from build123d import *

# Parameters (mm, degrees)
CUT_EXTRUDE1_START    = -16
CUT_EXTRUDE1_DEPTH    = 16
F_3_0MM_DOWEL_HOLE1_D = 3
CUT_EXTRUDE3_START    = -20
SKETCH17_R            = 5
SKETCH17_R_2          = 4
CUT_EXTRUDE3_DEPTH    = 1.5
CHAMFER2_SIZE         = 1
THREAD2_PITCH         = 1


with BuildPart() as part:
    # Sketch1 → Revolve1 (revolve)
    with BuildSketch(Plane.XY, mode=Mode.PRIVATE) as revolve1_sk:
        Polygon((0, 0), (0, 5), (45, 5), (45, 4), (60, 4), (60, 0), align=None)
    revolve(revolve1_sk.sketch.rotate(Axis((0, 0, 0), (1, 0, 0)), 90), axis=Axis((0, 0, 0), (1, 0, 0)))

    # Sketch2 → Cut-Extrude1 (cut)
    with BuildSketch(Plane.ZY.offset(CUT_EXTRUDE1_START)):
        with BuildLine():
            Line((-3, 4), (3, 4))
            ThreePointArc((3, 4), (0, 5), (-3, 4))
        make_face()
        with BuildLine():
            Line((3, -4), (-3, -4))
            ThreePointArc((-3, -4), (0, -5), (3, -4))
        make_face()
    extrude(amount=CUT_EXTRUDE1_DEPTH, mode=Mode.SUBTRACT)

    # Ø3.0mm Dowel Hole1 (through all)
    with Locations(Plane(origin=(0, 4, 0), x_dir=(1, 0, 0), z_dir=(0, 1, 0))):
        with Locations((10, 0)):
            Hole(F_3_0MM_DOWEL_HOLE1_D / 2)

    # Sketch17 → Cut-Extrude3 (cut)
    with BuildSketch(Plane(origin=(60, 0, 0), x_dir=(0, 0, -1), z_dir=(1, 0, 0)).offset(CUT_EXTRUDE3_START)):
        with Locations(Location((0, 0, 0), (0, 0, 180))):
            Circle(SKETCH17_R)
        with Locations(Location((0, 0, 0), (0, 0, 180))):
            Circle(SKETCH17_R_2, mode=Mode.SUBTRACT)
    extrude(amount=-CUT_EXTRUDE3_DEPTH, mode=Mode.SUBTRACT)

    # Chamfer2
    chamfer2_edges = [part.edges().sort_by_distance(p)[0] for p in [
        (40, 0, -5),
        (45, 0, -5),
    ]]
    chamfer(chamfer2_edges, length=CHAMFER2_SIZE - 0.0001)  # a hair under: the kernel refuses the full size

    # Thread2: the profile of Thread Profile2 profile screwed along a right-hand helix of 3 turns, 8 arcs to a turn; built about Z, then put on its axis
    thread2_z = Axis((0, 0, 0), (0, 0, 1))
    thread2_corners = [(5.0003, 0, -0.000173205), (5.0003, 0, 0.875173202), (4.458734125, 0, 0.562499999), (4.458734125, 0, 0.312499999)]
    with BuildLine(mode=Mode.PRIVATE) as thread2_profile:
        Line(thread2_corners[0], thread2_corners[1])
        Line(thread2_corners[1], thread2_corners[2])
        Line(thread2_corners[2], thread2_corners[3])
        Line(thread2_corners[3], thread2_corners[0])
    thread2_cap = Face(thread2_profile.wire())
    thread2_turn_angles = [0, 22.5, 45, 67.5, 90, 112.5, 135, 157.5, 180, 202.5, 225, 247.5, 270, 292.5, 315, 337.5, 360]
    thread2_turn_weights = [1, 0.9238795325112867, 1, 0.9238795325112867, 1, 0.9238795325112867, 1, 0.9238795325112867, 1, 0.9238795325112867, 1, 0.9238795325112867, 1, 0.9238795325112867, 1, 0.9238795325112867, 1]
    thread2_turn_rails = [Edge.make_bspline([Vector(p[0], p[1], 0).rotate(thread2_z, thread2_turn_angles[k]) / thread2_turn_weights[k] + Vector(0, 0, p[2] + THREAD2_PITCH * thread2_turn_angles[k] / 360) for k in range(17)], [0, 0, 0, 1, 1, 2, 2, 3, 3, 4, 4, 5, 5, 6, 6, 7, 7, 8, 8, 8], 2, thread2_turn_weights) for p in thread2_corners]
    thread2_turn_sides = [Face.make_surface_from_curves(thread2_turn_rails[p[0]], thread2_turn_rails[p[1]]) for p in [(0, 1), (1, 2), (2, 3), (3, 0)]]
    thread2 = Plane(origin=(44, 0, 0), x_dir=(0, 0, 1), z_dir=(-1, 0, 0)) * Solid(Shell([*[p.moved(Location((0, 0, THREAD2_PITCH * i))) for i in range(3) for p in thread2_turn_sides], thread2_cap, thread2_cap.rotate(thread2_z, 1080).moved(Location((0, 0, THREAD2_PITCH * 1080 / 360)))]))
    add(thread2, mode=Mode.SUBTRACT)


solid = part.part
Here's how the part is built. I have some questions about the finished solid (model axes, mm). A direction names the side the tool comes from. Give positions to 0.01 mm unless a question says otherwise; leave off trailing zeros. Order: outer loops, then holes, each group sorted by start corner. A loop starts at its lowest first (then second) coordinate and runs counter-clockwise, first axis right, second up. Notation, with made-up numbers: M 61.5,-24 L 101.5,-24 A34 ccw 101.5,6 Z; hole C -4,28 d2. An arc over 180 degrees is marked long. Answer as a JSON object with one key per item and string values. Group by question number.
1) On a 3-axis mill with a long thin cutter (end or side, diameter ignored), from which of +Z, -Z, +X, -X, +Y, -Y can I reach the whole of each face in a straight line? I mean faces 4 (the cylindrical face through (52.605, 3.905, -0.867)), 5 (the flat face through (16, -4.4, 0)), 6 (the flat face through (16, 4.4, 0)), 7 (the flat face through (0, 0, 0)), 8 (the cylindrical face through (39.26, 3.905, -0.867)). Say none if no direction works.
2) Please list where these lines run through material, in increasing order: L1, parallel to Y at x = 57.5, z = -0.25; L2, parallel to Z at x = 2, y = -3; L3, parallel to Z at x = 10, y = -0.5. Write a range as [from, to].
3) We'd pull the mould along Z, two halves only. Please class faces 1 (the cylindrical face through (11.5, -0.06, -0.07)), 2 (the flat face through (8, -4, 0)), 3 (the cylindrical face through (24, 0, -5)): pulls with the +Z half, pulls with the -Z half, needs draft (parallel to the pull), parting line crosses it, or undercut.
4) Suppose I cut it at A-A, the plane x = 10. Write out the boundary of the cut face in (y, z), plus the area to 3 significant figures.
5) Suppose I cut it at B-B, the plane x = 54.5. Write out the boundary of the cut face in (y, z).
6) I'm going to push flat-ended pins straight in: pin 1 Ø0.8 at (y, z) = (4.5, -1) entering from -X; pin 2 Ø2 at (x, z) = (19, -0.5) entering from +Y; pin 3 Ø2 at (x, z) = (41, -2) entering from +Y; pin 4 Ø4 at (x, z) = (12, 1.5) entering from +Y. Where does each tip first touch, or does it pass through?
7) Suppose I cut it at C-C, the plane x = 23.5. Write out the boundary of the cut face in (y, z).
Results found:
{
 "1": {"face 4": "+X", "face 5": "+Z, -Z, -X, -Y", "face 6": "+Z, -Z, -X, +Y", "face 7": "+Z, -Z, -X, +Y, -Y", "face 8": "none"},
 "2": {"L1": "[-3.99, 3.99]", "L2": "[-4, 4]", "L3": "[-4.97, -1.5], [1.5, 4.97]"},
 "3": {"face 1": "undercut", "face 2": "needs draft", "face 3": "parting line crosses it"},
 "4": {"outline": "M -4,-3 A5 ccw 4,-3 L 4,-1.5 L -4,-1.5 Z; M -4,1.5 L 4,1.5 L 4,3 A5 ccw -4,3 Z", "area": "46.4 mm²"},
 "5": {"outline": "C 0,0 d8"},
 "6": {"pin 1": "x = 16", "pin 2": "y = 5", "pin 3": "y = 4.83", "pin 4": "y = 4"},
 "7": {"outline": "C 0,0 d10"}
}
